Autodesk Inventor part; units mm, degrees
ref_plane "Arbeitsebene1" through (-73.4, -48.5, 0) normal (-1, 0, 0) x (0, 0, 1)
ref_plane "Arbeitsebene2" through (-42.4, -48.5, 0) normal (-1, 0, 0) x (0, 0, 1)
ref_plane "YZ Plane" through (0, 0, 0) normal (1, 0, 0) x (0, 1, 0)
sketch "Skizze3" plane through (0, 0, 0) normal (0, 0, 1) x (1, 0, 0)
  line L0 (0, 0) -> (-86, 0)
  line L1 (-86, 0) -> (-86, -66)
  line L2 (-86, -66) -> (0, -66)
  line L3 (0, -66) -> (0, 0)
  line L4 (-57.9, -33) -> (-86, -33) construction
  line L5 (-42.4, -48.5) -> (-73.4, -48.5) construction
  line L6 (-74.4, -48.5) -> (-72.4, -48.5) construction
  line L7 (-74.4, -46.9) -> (-72.4, -46.9)
  line L8 (-72.4, -50.1) -> (-74.4, -50.1)
  arc A0 (-74.4, -46.9) -> (-74.4, -50.1) centre (-74.4, -48.5) ccw
  arc A1 (-72.4, -50.1) -> (-72.4, -46.9) centre (-72.4, -48.5) ccw
  line L9 (-43.4, -48.5) -> (-41.4, -48.5) construction
  line L10 (-43.4, -50.1) -> (-41.4, -50.1)
  line L11 (-41.4, -46.9) -> (-43.4, -46.9)
  arc A2 (-43.4, -46.9) -> (-43.4, -50.1) centre (-43.4, -48.5) ccw
  arc A3 (-41.4, -50.1) -> (-41.4, -46.9) centre (-41.4, -48.5) ccw
  line L12 (-74.4, -19.1) -> (-72.4, -19.1)
  line L13 (-72.4, -15.9) -> (-74.4, -15.9)
  arc A4 (-74.4, -15.9) -> (-74.4, -19.1) centre (-74.4, -17.5) ccw
  arc A5 (-72.4, -19.1) -> (-72.4, -15.9) centre (-72.4, -17.5) ccw
  line L14 (-43.4, -15.9) -> (-41.4, -15.9)
  line L15 (-41.4, -19.1) -> (-43.4, -19.1)
  arc A6 (-43.4, -15.9) -> (-43.4, -19.1) centre (-43.4, -17.5) ccw
  arc A7 (-41.4, -19.1) -> (-41.4, -15.9) centre (-41.4, -17.5) ccw
  line L16 (-58.9, -33) -> (-56.9, -33) construction
  line L17 (-58.9, -44) -> (-56.9, -44)
  line L18 (-56.9, -22) -> (-58.9, -22)
  arc A8 (-58.9, -22) -> (-58.9, -44) centre (-58.9, -33) ccw
  arc A9 (-56.9, -44) -> (-56.9, -22) centre (-56.9, -33) ccw
  point P0 (-57.9, -48.5)
  dimension "d4" = 86
  dimension "d5" = 66
  dimension "d44" = 31
  dimension "d53" = 28.1
  dimension "d54" = 15.5
  dimension "d55" = 1.6
  dimension "d56" = 2
  dimension "d57" = 1.6
  dimension "d58" = 2
  dimension "d59" = 2
  dimension "d60" = 11
extrude "Extrusion3" add sketch "Skizze3" along normal blind 6 contours L3 L2 L1 L0 | L7 A1 L8 A0 | A2 L11 A3 L10 | A4 L13 A5 L12 | L14 A7 L15 A6 | A8 L18 A9 L17
sketch "Skizze4" plane through (0, -66, 0) normal (1, 0, 0) x (0, 0, -1)
  line L0 (0, 0) -> (-6, 0)
  line L1 (-3, 0) -> (-3, 70) construction
  line L2 (0, 66) -> (0, 0)
  line L3 (0, 66) -> (-6, 66)
  point P0 (-3, 60)
  point P1 (-3, 6)
  dimension "d10" = 6
  dimension "d11" = 6
hole "Bohrung1" at (0, -6, 3) at (0, -60, 3) direction (-1, 0, 0) diameter 3 depth 10 tip angle 118
thread "Gewinde2"
thread "Gewinde3"
sketch "Skizze5" plane through (0, 0, 6) normal (0, 0, 1) x (1, 0, 0)
  line L0 (0, -60) -> (-86, -60) construction
  line L1 (-86, 0) -> (-86, -66)
  line L2 (-70, -63.025) -> (-86, -63.025)
  line L3 (-86, -63.025) -> (-86, -56.975)
  line L4 (-86, -56.975) -> (-70, -56.975)
  line L5 (-70, -56.975) -> (-70, -63.025)
  line L6 (0, -66) -> (0, 0)
  line L7 (0, -33) -> (-86, -33) construction
  line L8 (-70, -2.975) -> (-86, -2.975)
  line L9 (-86, -2.975) -> (-86, -9.025)
  line L10 (-86, -9.025) -> (-70, -9.025)
  line L11 (-70, -9.025) -> (-70, -2.975)
  point P0 (0, -6)
  point P1 (-80, -60)
  point P2 (-70, -60)
  point P3 (-80, -6)
  point P4 (-86, -2.975)
  point P5 (-86, -9.025)
  dimension "d26" = 6
  dimension "d34" = 16
  dimension "d35" = 6.05
hole "Bohrung2" at (-80, -60, 6) at (-80, -6, 6) direction (0, 0, -1) diameter 3.3 depth 8.1
sketch "Skizze6" plane through (0, 0, 0) normal (0, 0, -1) x (-1, 0, 0)
  line L0 (86, -9.025) -> (70, -9.025)
  line L1 (70, -9.025) -> (70, -2.975)
  line L2 (70, -2.975) -> (86, -2.975)
  line L3 (86, -56.975) -> (70, -56.975)
  line L4 (70, -63.025) -> (86, -63.025)
  line L5 (70, -56.975) -> (70, -63.025)
  line L6 (86, 0) -> (86, -66)
  point P0 (0, 0)
  point P1 (80, -6)
extrude "Extrusion5" cut sketch "Skizze6" against normal blind 1
fillet "Rundung3" radius 2 4 edges at (0, -66, 3) (0, 0, 3) (-86, -66, 3) (-86, 0, 3)
fillet "Rundung4" radius 2 8 edges at (-86, -2.975, 0.5) (-86, -9.025, 0.5) (-70, -2.975, 0.5) (-70, -9.025, 0.5) (-86, -56.975, 0.5) (-86, -63.025, 0.5) (-70, -56.975, 0.5) (-70, -63.025, 0.5)
extrude "Extrusion6" cut sketch "Skizze3" along normal blind 10 contours L7 A1 L8 A0 | A2 L11 A3 L10 | A4 L13 A5 L12 | L14 A7 L15 A6 | A8 L18 A9 L17
ref_plane "Arbeitsebene1" through (-73.4, -48.5, 0) normal (-1, 0, 0) x (0, 0, 1)
ref_plane "Arbeitsebene2" through (-42.4, -48.5, 0) normal (-1, 0, 0) x (0, 0, 1)
equation "\"d54\" = 0.5 * d44"
equation "\"d57\" = d55"
properties part number "BT901_goteln20_23" material "Acryl"
The model under review builds one solid part; all positions refer to its coordinate system, in mm. A direction names the side the tool comes from. Coordinates: 2 decimals unless noted, no trailing zeros. Order: outer loops, then holes, each group sorted by start corner. A loop starts at its lowest first (then second) coordinate and runs counter-clockwise, first axis right, second up. Notation, with made-up numbers: (-8.75, 19) -> (41.25, 19) arc R20 cw to (41.25, 37) -> close; hole circle Ø10 at (81, 25). An arc over 180 degrees is marked (long way). Answer in a Markdown table with one row per item. Add a question column.
Item 1: We need section D-D on y = -33. Write out the cut boundary in (x, z), plus the area to 3 significant figures.
Item 2: We need section B-B on y = -17.5. Write out the cut boundary in (x, z), plus the area to 3 significant figures.
Item 3: We need section A-A on x = -80. Write out the cut boundary in (y, z) (3 decimals), plus the area to 3 significant figures.
Item 4: To check wall thickness, follow probe 1 along Y at (x, z) = (-80, 4.15); probe 2 along Y at (x, z) = (-8, 3); probe 3 along Z at (x, y) = (-6, -6). State the ranges of each line that lie inside material, in increasing order.
Item 5: Clearance check with a flat-ended pin moving along its axis: pin 1 (0.8 mm diameter, centred on y = -6, z = 0.5, fed in from -X). State where the tip first meets the part, or that it passes through.
Item 6: We need section C-C on x = -66. Write out the cut boundary in (y, z), plus the area to 3 significant figures.
Item 7: Machinability: for faces 1 (the cylindrical face through (-85.399, -56.405, 0.493)), 2 (the flat face through (-42, 0, 3)), 3 (the cylindrical face through (-39.8, -17.5, 3)), which of the approach directions +Z, -Z, +X, -X, +Y, -Y give a long, thin tool a straight path to every point of the face, cutting with its end or side? Answer none if there is none.
Item 8: Mouldability with a two-part tool opening along Y and no side actions: class faces 4 (the cylindrical face through (-70.601, -3.545, 0.493)), 5 (the flat face through (-44, -33, 0)), 6 (the cylindrical face through (-0.57, -0.6, 3.04)) as +Y half, -Y half, draft (parallel to the pull), parting line (faces both ways), or undercut.
Final values:
| question | item | result |
|---|---|---|
| 1 | outline | (-86, 0) -> (-69.9, 0) -> (-69.9, 6) -> (-86, 6) -> close; (-45.9, 0) -> (0, 0) -> (0, 6) -> (-45.9, 6) -> close |
| 1 | area | 372 mm2 |
| 2 | outline | (-86, 0) -> (-76, 0) -> (-76, 6) -> (-86, 6) -> close; (-70.8, 0) -> (-45, 0) -> (-45, 6) -> (-70.8, 6) -> close; (-39.8, 0) -> (0, 0) -> (0, 6) -> (-39.8, 6) -> close |
| 2 | area | 454 mm2 |
| 3 | outline | (-66, 0) -> (-63.025, 0) -> (-63.025, 1) -> (-61.65, 1) -> (-61.65, 6) -> (-66, 6) -> close; (-58.35, 1) -> (-56.975, 1) -> (-56.975, 0) -> (-9.025, 0) -> (-9.025, 1) -> (-7.65, 1) -> (-7.65, 6) -> (-58.35, 6) -> close; (-4.35, 1) -> (-2.975, 1) -> (-2.975, 0) -> (0, 0) -> (0, 6) -> (-4.35, 6) -> close |
| 3 | area | 351 mm2 |
| 4 | probe 1 | y = -66 to -61.65, -58.35 to -7.65, -4.35 to 0 |
| 4 | probe 2 | y = -66 to -61.5, -58.5 to -7.5, -4.5 to 0 |
| 4 | probe 3 | z = 0 to 1.5, 4.5 to 6 |
| 5 | pin 1 | stops at x = -70 |
| 6 | outline | (-66, 0) -> (-41.4, 0) -> (-41.4, 6) -> (-66, 6) -> close; (-24.6, 0) -> (0, 0) -> (0, 6) -> (-24.6, 6) -> close |
| 6 | area | 295 mm2 |
| 7 | face 1 | -Z, -X |
| 7 | face 2 | +Z, -Z, +X, -X, +Y |
| 7 | face 3 | +Z, -Z |
| 8 | face 4 | undercut |
| 8 | face 5 | draft |
| 8 | face 6 | +Y half |
